Geometry check sheet. Reference: drawing and pictorial views, mm from the part's lowest x, y, z. Give positions to 0.01 mm unless a question says otherwise; leave off trailing zeros. Order: outer loops, then holes, each group sorted by start corner. A loop starts at its lowest first (then second) coordinate and runs counter-clockwise, first axis right, second up.
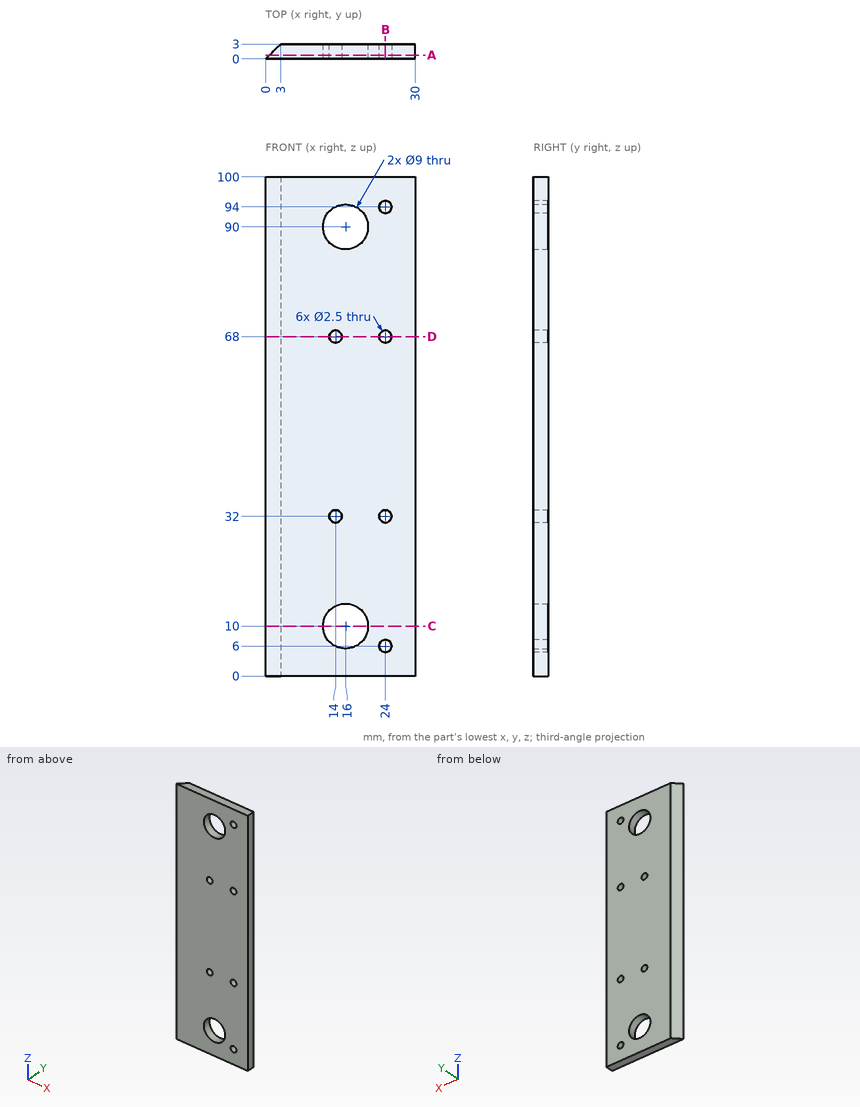
1) Section check C-C, the plane z = 10. Record the cut outline in (x, y).
Recorded:
outline: (0, 0) - (11.5, 0) - (11.5, 3) - (3, 3) - close; (20.5, 0) - (30, 0) - (30, 3) - (20.5, 3) - close
2) Section check D-D, the plane z = 68. Record the cut outline in (x, y).
Recorded:
outline: (0, 0) - (12.75, 0) - (12.75, 3) - (3, 3) - close; (15.25, 0) - (22.75, 0) - (22.75, 3) - (15.25, 3) - close; (25.25, 0) - (30, 0) - (30, 3) - (25.25, 3) - close
3) Material ranges on L1, parallel to X at y = 2.3, z = 32; L2, parallel to Z at x = 18, y = 1.3; L3, parallel to Z at x = 16, y = 1.65, recorded low to high.
Recorded:
L1: x = 2.3 to 12.75, 15.25 to 22.75, 25.25 to 30
L2: z = 0 to 5.97, 14.03 to 85.97, 94.03 to 100
L3: z = 0 to 5.5, 14.5 to 85.5, 94.5 to 100
4) Section check A-A, the plane y = 0.75. State how many separate pieces and enclosed holes the cut face has, then the cut area to 3 significant figures.
Recorded:
separate pieces: 1
enclosed holes: 8
area: 2,770 mm2
5) Section check B-B, the plane x = 24. Record the cut outline in (y, z), then the cut area to 3 significant figures.
Recorded:
outline: (0, 0) - (3, 0) - (3, 4.75) - (0, 4.75) - close; (0, 7.25) - (3, 7.25) - (3, 30.75) - (0, 30.75) - close; (0, 33.25) - (3, 33.25) - (3, 66.75) - (0, 66.75) - close; (0, 69.25) - (3, 69.25) - (3, 92.75) - (0, 92.75) - close; (0, 95.25) - (3, 95.25) - (3, 100) - (0, 100) - close
area: 270 mm2
